Check sheet for the modelled part. Datum: model origin and axes. Units: mm. Round coordinates to 2 decimals unless told otherwise and drop trailing zeros. Loops run counter-clockwise (first coordinate to the right, second up) from the corner with the lowest first, then second, coordinate; pieces in that order, holes last. Notation, with made-up numbers: M -7,26 L 5,26 A27 ccw 5,65 Z; hole C -4,87.5 d3. An arc over 180 degrees is marked long. Write item = value, one per line. Start each with the question number.
(1) Cross-section at C-C on x = 25. Record the boundary of the cut face in (y, z), plus the area to 3 significant figures.
(2) Scan lines: L1, parallel to Y at x = 0, z = 1.5; L2, parallel to X at y = -1, z = 0.7; L3, parallel to X at y = 15.5, z = 2.4. Record each from-to range of solid material in increasing order. Write a range as from..to.
(3) Cross-section at D-D on z = 2. State how many separate pieces and enclosed holes the cut face has, plus the area to 3 significant figures.
(4) Cross-section at A-A on y = 0. Record the boundary of the cut face in (x, z).
(5) Go/stop test with flat-tipped pins: P1, Ø0.9, axis at x = 0, z = 2, coming from the -Y side; P2, Ø9, axis at x = 0, y = 0, coming from the -Z side; P3, Ø12, axis at x = 3, y = 25.5, coming from the -Z side; P4, Ø1, axis at y = 42, z = 0.5, coming from the -X side. Record where each tip stops, or that it passes through.
from build123d import *

# Parameters (mm, degrees)
SKETCH1_R               = 52.5
BOSS_EXTRUDE1_DEPTH     = 3
RIB_START               = -47.5
RIB_SLOT_OUTLINE_W      = 3.2
RIB_SLOT_OUTLINE_H      = 3
RIB_SLOT_DEPTH          = 5
RIB_START_2             = -32.5
RIB_SLOT_2_OUTLINE_W    = 3.2
RIB_SLOT_2_OUTLINE_H    = 3
RIB_SLOT_2_DEPTH        = 5
RIB_SLOT_PATTERN_COUNT  = 4
ANTENNA_CLEARANCE_REACH = 76.307
SKETCH3_R               = 5


# Read off the part's stored shape, not the designer's step: rib slot
with BuildPart() as part:
    # Sketch1 → Boss-Extrude1 (new body)
    with BuildSketch(Plane.XY):
        with Locations(Location((0, 0, 0), (0, 0, 180))):
            Circle(SKETCH1_R)
    extrude(amount=BOSS_EXTRUDE1_DEPTH)

    # rib slot outline → rib slot (cut)
    with BuildSketch(Plane(origin=(0, 0, 0), x_dir=(1, 0, 0), z_dir=(0, 1, 0)).offset(RIB_START)):
        with Locations((0, -1.5)):
            Rectangle(RIB_SLOT_OUTLINE_W, RIB_SLOT_OUTLINE_H)
    rib_slot = extrude(amount=RIB_SLOT_DEPTH, mode=Mode.SUBTRACT)

    # rib slot 2 outline → rib slot 2 (cut)
    with BuildSketch(Plane(origin=(0, 0, 0), x_dir=(1, 0, 0), z_dir=(0, 1, 0)).offset(RIB_START_2)):
        with Locations((0, -1.5)):
            Rectangle(RIB_SLOT_2_OUTLINE_W, RIB_SLOT_2_OUTLINE_H)
    rib_slot_2 = extrude(amount=RIB_SLOT_2_DEPTH, mode=Mode.SUBTRACT)

    # rib slot pattern: rib slot, rib slot 2 ×4 about axis
    rib_slot_pattern_axis = Axis((0, 0, 0), (0, 0, 1))
    add([rib_slot.rotate(rib_slot_pattern_axis, i * 360 / RIB_SLOT_PATTERN_COUNT) for i in range(1, RIB_SLOT_PATTERN_COUNT)], mode=Mode.SUBTRACT)
    add([rib_slot_2.rotate(rib_slot_pattern_axis, i * 360 / RIB_SLOT_PATTERN_COUNT) for i in range(1, RIB_SLOT_PATTERN_COUNT)], mode=Mode.SUBTRACT)

    # Sketch3 → antenna clearance (cut, up to next)
    with BuildSketch(Plane.XY.offset(3), mode=Mode.PRIVATE) as antenna_clearance_sk1:
        Circle(SKETCH3_R)
    antenna_clearance_tool1 = extrude(antenna_clearance_sk1.sketch, amount=-ANTENNA_CLEARANCE_REACH, mode=Mode.PRIVATE) & part.part
    # Sketch3 → antenna clearance (cut, up to next)
    with BuildSketch(Plane.XY.offset(3), mode=Mode.PRIVATE) as antenna_clearance_sk2:
        with BuildLine():
            Line((-21, 24), (-21, 16))
            ThreePointArc((-21, 16), (-25, 12), (-29, 16))
            Line((-29, 16), (-29, 24))
            ThreePointArc((-29, 24), (-25, 28), (-21, 24))
        make_face()
    antenna_clearance_tool2 = extrude(antenna_clearance_sk2.sketch, amount=-ANTENNA_CLEARANCE_REACH, mode=Mode.PRIVATE) & part.part
    # Sketch3 → antenna clearance (cut, up to next)
    with BuildSketch(Plane.XY.offset(3), mode=Mode.PRIVATE) as antenna_clearance_sk3:
        with BuildLine():
            Line((21, 24), (21, 16))
            ThreePointArc((21, 16), (25, 12), (29, 16))
            Line((29, 16), (29, 24))
            ThreePointArc((29, 24), (25, 28), (21, 24))
        make_face()
    antenna_clearance_tool3 = extrude(antenna_clearance_sk3.sketch, amount=-ANTENNA_CLEARANCE_REACH, mode=Mode.PRIVATE) & part.part
    add(antenna_clearance_tool1.solids().sort_by_distance((0, 0, 3))[0], mode=Mode.SUBTRACT)
    add(antenna_clearance_tool2.solids().sort_by_distance((-25, 20, 3))[0], mode=Mode.SUBTRACT)
    add(antenna_clearance_tool3.solids().sort_by_distance((25, 20, 3))[0], mode=Mode.SUBTRACT)


solid = part.part
Result:
q1.outline = M -46.17,0 L 12,0 L 12,3 L -46.17,3 Z; M 28,0 L 46.17,0 L 46.17,3 L 28,3 Z
q1.area = 229 mm^2
q2.L1 = -52.5..-47.5, -42.5..-32.5, -27.5..-5, 5..27.5, 32.5..42.5, 47.5..52.5
q2.L2 = -52.49..-47.5, -42.5..-32.5, -27.5..-4.9, 4.9..27.5, 32.5..42.5, 47.5..52.49
q2.L3 = -50.16..-28.97, -21.03..21.03, 28.97..50.16
q3.separate_pieces = 1
q3.enclosed_holes = 11
q3.area = 8,220 mm^2
q4.outline = M -52.5,0 L -47.5,0 L -47.5,3 L -52.5,3 Z; M -42.5,0 L -32.5,0 L -32.5,3 L -42.5,3 Z; M -27.5,0 L -5,0 L -5,3 L -27.5,3 Z; M 5,0 L 27.5,0 L 27.5,3 L 5,3 Z; M 32.5,0 L 42.5,0 L 42.5,3 L 32.5,3 Z; M 47.5,0 L 52.5,0 L 52.5,3 L 47.5,3 Z
q5.P1 = -52.5
q5.P2 = through
q5.P3 = 0
q5.P4 = -32.16
